Here's how the part is built. I have some questions about the finished solid (model axes, mm). A direction names the side the tool comes from. Coordinates: 2 decimals unless noted, no trailing zeros. Write each loop counter-clockwise with the first axis right and the second up, starting at its lowest first coordinate (ties: lowest second). Pieces come first, ordered by that corner, then holes.
Item 1: I want a section at A-A (z = 48). Please give me the cut outline in (x, y).
Item 2: I want a section at B-B (x = -91.5). Please give me the cut outline in (y, z).
Item 3: Please list where these lines run through material, in increasing order: line 1 (Z direction, x = -35.5, y = -9.75); line 2 (Z direction, x = -107, y = -12.75); line 3 (Z direction, x = -81.5, y = -9.5).
Item 4: For faces 1 (the face through (102.506, -12, -71)), 2 (the face through (22.506, -12, -82)), 3 (the face through (-158.084, -12.325, 38.793)), 4 (the face through (69.41, -12.32, -126.76)), 5 (the face through (-69, -12, 65.689)), which set-ups out of +Z, -Z, +X, -X, +Y, -Y let a thin tool reach every point of the face, with its end or its side?
Item 5: I'm going to push flat-ended pins straight in: P1, Ø7.5, axis at y = -6.5, z = -97, coming from the -X side; P2, Ø5, axis at y = -10, z = -22, coming from the +X side; P3, Ø2, axis at x = 20, z = -80.5, coming from the -Y side; P4, Ø7.5, axis at x = -59, y = -7, coming from the +Z side. Where does each tip first touch, or does it pass through?
Item 6: I want a section at D-D (z = -80). Please give me the cut outline in (x, y).
Item 7: If we mould it in two halves opening along X, with no side actions, what happens to faces 6 (the face through (-110.224, -12.325, 25.127)), 7 (the face through (-89, -12, 10.689)), 8 (the face through (134.166, -12, 39)), 9 (the face through (-32.97, -12.32, 57.54))? For each: pulls with the +X half, pulls with the -X half, needs draft (parallel to the pull), parting line crosses it, or undercut.
Item 8: I want a section at C-C (y = -4.75). Count the separate pieces of the cut face and the enclosed holes in it, and give its area (3 significant figures).
from build123d import *

# Parameters (mm, degrees)
F0_R     = 14.959445
F0_R_2   = 7.087313
F1_DEPTH = 25
F2_R     = 35


with BuildPart() as f1:
    # F0 (on Front) → F1 (new body)
    with BuildSketch(Plane.XZ):
        with BuildLine():
            add(Edge.make_bspline(
                [(-45.392299, 10.688528), (22.505625, 10.688528), (22.505625, 10.688528), (22.505625, -51.399426)],
                knots=[0, 0, 0, 0, 92.005663, 92.005663, 92.005663, 92.005663], degree=3))
            Line((22.505625, -51.399426), (22.505625, -113.487379))
            ThreePointArc((22.505625, -113.487379), (62.505625, -153.487379), (102.505625, -113.487379))
            Line((102.505625, -113.487379), (102.505625, -26.389777))
            add(Edge.make_bspline(
                [(134.16557, 14.047909), (102.505625, 14.534711), (102.505625, 14.216591), (102.505625, -26.389777)],
                knots=[0, 0, 0, 0, 51.357167, 51.357167, 51.357167, 51.357167], degree=3))
            Line((134.16557, 14.047909), (134.16557, 99.047909))
            Line((134.16557, 99.047909), (22.505625, 99.047909))
            add(Edge.make_bspline(
                [(22.505625, 99.047909), (22.505625, 64.501319), (22.505625, 65.688528), (-9.330841, 65.688528)],
                knots=[0, 0, 0, 0, 46.113002, 46.113002, 46.113002, 46.113002], degree=3))
            Line((-9.330841, 65.688528), (-130.590424, 65.688528))
            ThreePointArc((-130.590424, 65.688528), (-158.090424, 38.188528), (-130.590424, 10.688528))
            Line((-130.590424, 10.688528), (-45.392299, 10.688528))
        make_face()
        with Locations((62.505625, -113.487379)):
            Circle(F0_R, mode=Mode.SUBTRACT)
        with Locations((-103.143071, 24.815377)):
            Circle(F0_R_2, mode=Mode.SUBTRACT)
        with Locations((-36.778194, 24.815377)):
            Circle(F0_R_2, mode=Mode.SUBTRACT)
        with Locations((-103.143071, 51.561678)):
            Circle(F0_R_2, mode=Mode.SUBTRACT)
        with Locations((-36.778194, 51.561678)):
            Circle(F0_R_2, mode=Mode.SUBTRACT)
    extrude(amount=F1_DEPTH)

    # F2
    f2_edges = [f1.edges().sort_by_distance(p)[0] for p in [
        (134.16557, -12.5, 99.047909),
    ]]
    fillet(f2_edges, radius=F2_R)


solid = f1.part
Answer:
1. outline: (-156.28, -25) - (-109.27, -25) - (-109.27, 0) - (-156.28, 0) - close; (-97.02, -25) - (-42.91, -25) - (-42.91, 0) - (-97.02, 0) - close; (-30.65, -25) - (134.17, -25) - (134.17, 0) - (-30.65, 0) - close
2. outline: (-25, 10.69) - (0, 10.69) - (0, 65.69) - (-25, 65.69) - close
3. line 1: z = 10.68 to 17.84, 31.79 to 44.59, 58.53 to 65.69
3. line 2: z = 10.69 to 18.87, 30.76 to 45.62, 57.51 to 65.69
3. line 3: z = 10.69 to 65.69
4. face 1: -Z, +X, +Y, -Y
4. face 2: -Z, -X, +Y, -Y
4. face 3: -X, +Y, -Y
4. face 4: +Y, -Y
4. face 5: +Z, -X, +Y, -Y
5. P1: stops at x = 22.51
5. P2: stops at x = 102.51
5. P3: passes through
5. P4: stops at z = 65.69
6. outline: (22.51, -25) - (102.51, -25) - (102.51, 0) - (22.51, 0) - close
7. face 6: undercut
7. face 7: needs draft
7. face 8: pulls with the +X half
7. face 9: undercut
8. separate pieces: 1
8. enclosed holes: 5
8. area: 30,500 mm2
